```python
from build123d import *

# Parameters (mm, degrees)
F1_R     = 21
F1_R_2   = 19
F3_DEPTH = 100
F4_DEPTH = 50
F7_DEPTH = 25


with BuildPart() as f2:
    # F2: sweep along a path in F0
    with BuildLine(Plane.YZ) as f2_path:
        ThreePointArc((0, -80), (-56.5685424949, -56.5685424949), (-80, 0))
    # F1 (on Top) → F2 (sweep)
    with BuildSketch(Plane.XY):
        with Locations((0, -80.018363893)):
            Circle(F1_R)
        with Locations((0, -80.018363893)):
            Circle(F1_R_2, mode=Mode.SUBTRACT)
    sweep(path=f2_path.line)

    # F3 (add): a face of the model
    f3_faces = [f2.faces().sort_by_distance(p)[0] for p in [
        (-20.4060303038, -80.018363893, 0),
    ]]
    extrude(f3_faces, amount=F3_DEPTH)

    # F4 (add): a face of the model
    f4_faces = [f2.faces().sort_by_distance(p)[0] for p in [
        (-20.4060303038, 0, -80.018363893),
    ]]
    extrude(f4_faces, amount=F4_DEPTH)

    # F6 (on face) → F7 (cut, symmetric)
    with BuildSketch(Plane(origin=(-4.1820983055, 0, -79.7991894081), x_dir=(0.9986295348, 0, -0.0523359562), z_dir=(0.0523359562, 0, 0.9986295348))):
        Polygon((58.3756751827, 50), (23.1878375913, 50), (10.5211709247, 50), (22.799627015, -50), (58.3756751827, -50), align=None)
    extrude(amount=F7_DEPTH, both=True, mode=Mode.SUBTRACT)


solid = f2.part
```
Source: CAD feature listing. Evaluate the final solid. Frame: model axes, mm. A direction names the side the tool comes from. Give positions to 0.01 mm unless a question says otherwise; leave off trailing zeros. Loops run counter-clockwise (first coordinate to the right, second up) from the corner with the lowest first, then second, coordinate; pieces in that order, holes last. Notation, with made-up numbers: M 45,-38 L 96,-38 A16 ccw 96,-24 Z; hole C -36,34.25 d9. An arc over 180 degrees is marked long. Put each result on its own line as item: value.
Q1. Reachability of faces 5 (the cylindrical face through (-21, 25, -80)), 6 (the cylindrical face through (-15.48, -94.21, 49.3)), 7 (the flat face through (11, -96, 100)) from +Z, -Z, +X, -X, +Y, -Y: full face, straight path, thin tool, end or side. Return the list, or none.
Response values:
face 5: +Y
face 6: +Z
face 7: +Z, +X, -X, +Y, -Y
Q2. Line query: probe 1 along Y at (x, z) = (0, 27.5); probe 2 along X at (y, z) = (-93, -8). Output: solid intervals per line, ascending. Write a range as [from, to].
Response values:
probe 1: y = [-101.02, -99.02], [-61.02, -59.02]
probe 2: x = [-16.23, -13.54], [13.54, 16.23]
Q3. Pin query (flat end, axial travel): P1, Ø10, axis at x = -13.5, y = 20, coming from the -Z side; P2, Ø3, axis at y = -70, z = -16.5, coming from the +X side; P3, Ø1.5, axis at x = 0, y = 9.5, coming from the -Z side; P4, Ø2, axis at x = 6.5, y = -48.5, coming from the +Z side. Return the tip coordinate at first contact, or that it passes through.
Response values:
P1: stops at z = -99.22
P2: stops at x = 19.94
P3: stops at z = -101.02
P4: stops at z = -33.89
Q4. Mould query, pull axis X, two halves, no side actions, for faces 1 (the cylindrical face through (-19, 25, -80)), 2 (the flat face through (14.536, -10.878, -66.494)), 3 (the cylindrical face through (-15.08, -68.46, 49.3)), 4 (the flat face through (-19.4, 50, -78.4)). Classes: released by +X, released by -X, zero draft, split by the parting line, or undercut.
Response values:
face 1: undercut
face 2: released by +X
face 3: undercut
face 4: zero draft
Q5. Section B-B (x = -13.5). Return the cut outline in (y, z), and give its area (3 significant figures).
Response values:
outline: M -96.1,0 A96.1 ccw 0,-96.1 L 50,-96.1 L 50,-93.39 L 0,-93.39 A93.39 cw -93.39,0 L -93.39,100 L -96.1,100 Z; M -66.65,0 A66.65 ccw 0,-66.65 L 50,-66.65 L 50,-63.93 L 0,-63.93 A63.93 cw -63.93,0 L -63.93,100 L -66.65,100 Z
area: 1,500 mm²
Q6. Section D-D (y = 28.5). Return the cut outline in (x, z), and give its area (3 significant figures).
Response values:
outline: M 7.97,-99.45 L 8.08,-97.21 A19 cw long 9.84,-63.76 L 9.95,-61.53 A21 ccw long Z
area: 163 mm²
Q7. Section A-A (x = 0). Return the cut outline in (y, z), and give its area (3 significant figures).
Response values:
outline: M -101.02,0 A101.02 ccw 0,-101.02 L 50,-101.02 L 50,-99.02 L 0,-99.02 A99.02 cw -99.02,0 L -99.02,100 L -101.02,100 Z; M -61.02,0 A61.02 ccw 0,-61.02 L 50,-61.02 L 50,-59.02 L 0,-59.02 A59.02 cw -59.02,0 L -59.02,100 L -61.02,100 Z
area: 1,100 mm²
Q8. Section C-C (z = 51). Return the cut outline in (x, y), and give its area (3 significant figures).
Response values:
outline: C 0,-80.02 d42; hole C 0,-80.02 d38
area: 251 mm²
